Could you check a few things on this model? Use its own coordinates, in mm. Coordinates: 2 decimals unless noted, no trailing zeros. Loops run counter-clockwise (first coordinate to the right, second up) from the corner with the lowest first, then second, coordinate; pieces in that order, holes last. Notation, with made-up numbers: (21.25, -22.75) -> (71.25, -22.75) arc R25 ccw to (71.25, 13.25) -> close; hole circle Ø10 at (23, 66.5). An arc over 180 degrees is marked (long way). One line per question, with ' | ' between items. Start each with the question number.
(1) Suppose I cut it at B-B (z = -189.5). Please give me the cut outline in (x, y) (3 decimals).
(2) Suppose I cut it at A-A (y = -37.95). Please give me the cut outline in (x, z) (1 decimal), plus the area to 3 significant figures.
(3) Suppose I cut it at C-C (y = -138). Please give me the cut outline in (x, z) (3 decimals), plus the area to 3 significant figures.
(4) If I drill on line 1 along Z through (x, y) = (1.8, -133.2) (1 decimal); line 2 along Y through (x, z) = (1.3, -219) (3 decimals); line 3 along Y through (x, z) = (2.4, -214.5) (3 decimals), over which ranges is the centre line in solid material (lowest first)?
(5) Suppose I cut it at D-D (x = 1.25). Give the number of separate pieces and of enclosed holes in the cut face, plus the area to 3 significant figures.
(6) If we mould it in two halves opening along Z, with no side actions, what happens to faces 1 (the face through (1.57, -135.06, -226.74)), 2 (the face through (1.57, -22.65, -248.09)), 3 (the face through (1.61, -15.1, -257.94)), 4 (the face through (1.61, -14.81, -167.5))? For each: pulls with the +Z half, pulls with the -Z half, needs draft (parallel to the pull), parting line crosses it, or undercut.
(7) I'm going to push flat-ended pins straight in: pin 1 Ø3 at (y, z) = (-47.475, -250.675) entering from -X; pin 2 Ø1 at (x, y) = (1, -141.5) entering from +Z. Where does each tip first touch, or does it pass through?
Autodesk Inventor part; units mm, degrees
ref_plane "YZ Plane" through (0, 0, 0) normal (1, 0, 0) x (0, 1, 0)
ref_plane "XZ Plane" through (0, 0, 0) normal (0, 1, 0) x (-1, 0, 0)
ref_plane "XY Plane" through (0, 0, 0) normal (0, 0, 1) x (1, 0, 0)
sketch "Sketch1" plane through (0, 0, 0) normal (1, 0, 0) x (0, 1, 0)
  line L0 (0, 0) -> (101.6, 0)
  line L1 (101.6, 0) -> (101.6, -152.4)
  line L2 (101.6, -152.4) -> (0, -152.4)
  line L3 (0, -152.4) -> (0, 0)
  circle A0 centre (50.8, -28.575) radius 14.2875
  circle A1 centre (50.8, -60.325) radius 6.35
  circle A2 centre (50.8, -92.075) radius 6.35
  circle A3 centre (50.8, -123.825) radius 14.2875
  line L4 (50.8, -28.575) -> (50.8, -123.825) construction
  circle A4 centre (88.9, -12.7) radius 2.65
  circle A5 centre (88.9, -38.1) radius 2.65
  circle A6 centre (88.9, -63.5) radius 2.65
  circle A7 centre (88.9, -88.9) radius 2.65
  circle A8 centre (88.9, -114.3) radius 2.65
  circle A9 centre (88.9, -139.7) radius 2.65
  circle A10 centre (12.7, -12.7) radius 2.65
  circle A11 centre (12.7, -38.1) radius 2.65
  circle A12 centre (12.7, -63.5) radius 2.65
  circle A13 centre (12.7, -88.9) radius 2.65
  circle A14 centre (12.7, -114.3) radius 2.65
  circle A15 centre (12.7, -139.7) radius 2.65
  line L5 (76.2, -152.4) -> (76.2, -508.635)
  line L6 (25.4, -187.175) -> (25.4, -152.4)
  circle A16 centre (50.8, -212.575) radius 6.35
  line L7 (50.8, -212.575) -> (-444.4159, 282.6409) construction
  line L8 (50.8, -212.575) -> (751.141, -212.575) construction
  line L9 (-161.775, -263.375) -> (-9.375, -263.375)
  line L10 (-9.375, -263.375) -> (-9.375, -161.775)
  line L11 (-9.375, -161.775) -> (-161.775, -161.775)
  circle A17 centre (-133.2, -212.575) radius 14.2875
  circle A18 centre (-101.45, -212.575) radius 6.35
  circle A19 centre (-69.7, -212.575) radius 6.35
  circle A20 centre (-37.95, -212.575) radius 14.2875
  line L12 (-133.2, -212.575) -> (-37.95, -212.575) construction
  circle A21 centre (-149.075, -250.675) radius 2.65
  circle A22 centre (-123.675, -250.675) radius 2.65
  circle A23 centre (-98.275, -250.675) radius 2.65
  circle A24 centre (-72.875, -250.675) radius 2.65
  circle A25 centre (-47.475, -250.675) radius 2.65
  circle A26 centre (-22.075, -250.675) radius 2.65
  circle A27 centre (-149.075, -174.475) radius 2.65
  circle A28 centre (-123.675, -174.475) radius 2.65
  circle A29 centre (-98.275, -174.475) radius 2.65
  circle A30 centre (-72.875, -174.475) radius 2.65
  circle A31 centre (-47.475, -174.475) radius 2.65
  circle A32 centre (-22.075, -174.475) radius 2.65
  line L13 (-9.375, -237.975) -> (346.86, -237.975)
  line L14 (25.4, -187.175) -> (-9.375, -187.175)
  circle A33 centre (50.8, -212.575) radius 6.35
  line L15 (50.8, -212.575) -> (50.8, -912.916) construction
  line L16 (76.2, -237.975) -> (346.86, -237.975)
  line L17 (76.2, -508.635) -> (76.2, -237.975)
  line L18 (-161.775, -161.775) -> (-161.775, -263.375)
  circle A34 centre (50.8, -28.575) radius 25.4 construction
  circle A35 centre (50.8, -28.575) radius 38.1
  circle A36 centre (82.55, -28.575) radius 2.65
  circle A37 centre (19.05, -28.575) radius 2.65
  line L19 (88.9, -28.575) -> (88.9, -47.625) construction
  line L20 (88.9, -47.625) -> (101.6, -47.625) construction
  line L21 (101.6, -47.625) -> (101.6, -66.675) construction
  spline S0 degree 3 poles (88.9, -28.575) (88.9, -47.625) (101.6, -47.625) (101.6, -66.675) knots 1 1 1 1 2 2 2 2
  line L22 (12.7, -28.575) -> (12.7, -47.625) construction
  line L23 (12.7, -47.625) -> (0, -47.625) construction
  line L24 (0, -47.625) -> (0, -66.675) construction
  spline S1 degree 3 poles (12.7, -28.575) (12.7, -47.625) (0, -47.625) (0, -66.675) knots 1 1 1 1 2 2 2 2
  spline S2 degree 3 poles (-133.2, -174.475) (-114.15, -174.475) (-114.15, -161.775) (-95.1, -161.775) knots 1 1 1 1 2 2 2 2
  line L25 (-133.2, -174.475) -> (-114.15, -174.475) construction
  line L26 (-114.15, -174.475) -> (-114.15, -161.775) construction
  line L27 (-114.15, -161.775) -> (-95.1, -161.775) construction
  circle A38 centre (-133.2, -212.575) radius 38.1
  circle A39 centre (-133.2, -180.825) radius 2.65
  spline S3 degree 3 poles (-133.2, -250.675) (-114.15, -250.675) (-114.15, -263.375) (-95.1, -263.375) knots 1 1 1 1 2 2 2 2
  line L28 (-133.2, -250.675) -> (-114.15, -250.675) construction
  line L29 (-114.15, -250.675) -> (-114.15, -263.375) construction
  line L30 (-114.15, -263.375) -> (-95.1, -263.375) construction
  circle A40 centre (-133.2, -244.325) radius 2.65
  point P0 (101.6, -76.2)
  point P1 (50.8, -76.2)
  point P2 (50.8, -152.4)
  point P3 (-85.575, -263.375)
  point P4 (-85.575, -212.575)
  point P5 (-9.375, -212.575)
  point P6 (63.5, -470.535)
  point P7 (0, -66.675)
  point P8 (-126.2384, -251.347)
  point P9 (-121.9095, -252.6512)
  dimension "d32" = 76.2
  dimension "d0" = 101.6
  dimension "d1" = 152.4
  dimension "d2" = 28.575
  dimension "d3" = 12.7
  dimension "d4" = 12.7
  dimension "d5" = 28.575
  dimension "d6" = 31.75
  dimension "d7" = 31.75
  dimension "d8" = 31.75
  dimension "d9" = 5.3
  dimension "d10" = 12.7
  dimension "d11" = 12.7
  dimension "d14" = 25.4
  dimension "d17" = 76.2
  dimension "d22" = 12.7
  dimension "d24" = 184
  dimension "d25" = 25.4
  dimension "d26" = 50.8
  dimension "d27" = 135
  dimension "d31" = 50.8
  dimension "d33" = 31.75
  dimension "d34" = 31.75
  dimension "d35" = 19.05
  dimension "d36" = 19.05
  dimension "d39" = 90
  dimension "d41" = 31.75
extrude "Extrusion1" add sketch "Sketch1" along normal blind 3.175 contours L10 L9 S3 A22 A38 A28 S2 L11 | A28 A38 S2 | S3 A22 A38 | A38 A28 A22 L18 | L18 A38 | A28 A38 S2 | S3 A38 A22 | A28 A38 | A22 A38
fillet "Fillet3" radius 19.05 2 edges at (1.5875, -9.375, -161.775) (1.5875, -9.375, -263.375)
sketch "Sketch3" plane through (3.175, 0, 0) normal (1, 0, 0) x (0, 0, -1)
  line L0 (244.325, -9.375) -> (180.825, -9.375)
  line L1 (212.575, -9.375) -> (212.575, -15.471)
  circle A0 centre (212.575, -15.471) radius 2.667
  point P0 (0, 0)
  dimension "d43" = 6.096
  dimension "d44" = 5.334
extrude "Extrusion2" cut sketch "Sketch3" against normal blind 25.4
equation "\"d7\" = d6"
equation "\"d8\" = d7"
properties part number "L1Plate" material "Aluminum 6061"
Checks:
1) outline: (0, -163.518) -> (3.175, -163.518) -> (3.175, -9.375) -> (0, -9.375) -> close
2) outline: (0, -263.4) -> (3.2, -263.4) -> (3.2, -226.9) -> (0, -226.9) -> close; (0, -198.3) -> (3.2, -198.3) -> (3.2, -161.8) -> (0, -161.8) -> close | area: 232 mm^2
3) outline: (0, -250.371) -> (3.175, -250.371) -> (3.175, -226.032) -> (0, -226.032) -> close; (0, -199.118) -> (3.175, -199.118) -> (3.175, -174.779) -> (0, -174.779) -> close | area: 155 mm^2
4) line 1: z = -250.7 to -247, -241.7 to -226.9, -198.3 to -183.5, -178.2 to -174.5 | line 2: y = -170.754 to -145.961, -120.439 to -50.711, -25.189 to -9.375 | line 3: y = -171.251 to -147.357, -119.043 to -107.501, -95.399 to -75.751, -63.649 to -52.107, -23.793 to -17.317, -13.625 to -9.375
5) separate pieces: 1 | enclosed holes: 15 | area: 12,400 mm^2
6) face 1: undercut | face 2: undercut | face 3: pulls with the -Z half | face 4: pulls with the +Z half
7) pin 1: passes through | pin 2: stops at z = -175.28
